from build123d import *

# Parameters (mm, degrees)
SKETCH_1_W               = 5
SKETCH_1_H               = 3.2
SKETCH_2_OUTSIDE_W       = 14.9
SKETCH_2_OUTSIDE_H       = 14.9
CUT_EXTRUDE_1_DEPTH      = 3.2
SKETCH_3_R               = 1.5
CUT_EXTRUDE_2_DEPTH      = 1
CUT_EXTRUDE_2_DEPTH_BACK = 4.2
CHAMFER_1_SIZE           = 0.4


with BuildPart() as part:
    # Эскиз1 → Повернуть1 (revolve)
    with BuildSketch(Plane(origin=(0, 0, 0), x_dir=(1, 0, 0), z_dir=(0, 1, 0))):
        with Locations((-2.5, 1.6)):
            Rectangle(SKETCH_1_W, SKETCH_1_H)
    revolve(axis=Axis((0, 0, 0), (0, 0, -1)))

    # Эскиз2 outside → Вырез-Вытянуть1 (cut)
    with BuildSketch(Plane.XY):
        Rectangle(SKETCH_2_OUTSIDE_W, SKETCH_2_OUTSIDE_H)
        Polygon((3, -1.732050808), (3, 1.732050808), (0, 3.464101615), (-3, 1.732050808), (-3, -1.732050808), (0, -3.464101615), align=None, mode=Mode.SUBTRACT)
    extrude(amount=-CUT_EXTRUDE_1_DEPTH, mode=Mode.SUBTRACT)

    # Эскиз3 → Вырез-Вытянуть2 (cut, two sides)
    with BuildSketch(Plane.XY) as cut_extrude_2_sk:
        Circle(SKETCH_3_R)
    extrude(amount=CUT_EXTRUDE_2_DEPTH, mode=Mode.SUBTRACT)
    extrude(cut_extrude_2_sk.sketch, amount=-CUT_EXTRUDE_2_DEPTH_BACK, mode=Mode.SUBTRACT)

    # Эскиз4 → Вырез-Повернуть1 (revolve, cut)
    with BuildSketch(Plane(origin=(0, 0, 0), x_dir=(0, 0, -1), z_dir=(1, 0, 0))):
        Polygon((0, 2.8), (0.383419246, 3.464101615), (0, 3.464101615), align=None)
        Polygon((3.2, 2.8), (2.816580754, 3.464101615), (3.2, 3.464101615), align=None)
    revolve(axis=Axis((0, 0, 0), (0, 0, -1)), mode=Mode.SUBTRACT)

    # Фаска1
    chamfer_1_edges = [part.edges().sort_by_distance(p)[0] for p in [
        (-1.5, 0, -3.2),
        (-1.5, 0, 0),
    ]]
    chamfer(chamfer_1_edges, length=CHAMFER_1_SIZE)


solid = part.part
Source: CAD feature listing. Evaluate the final solid. Frame: model axes, mm. Round coordinates to 2 decimals unless told otherwise and drop trailing zeros. Order: outer loops, then holes, each group sorted by start corner. A loop starts at its lowest first (then second) coordinate and runs counter-clockwise, first axis right, second up. Notation, with made-up numbers: (66, -21.75) - (104, -21.75) arc R18 cw to (104, -5.75) - close; hole circle Ø11 at (10, 21). An arc over 180 degrees is marked (long way). Use a Markdown table: item, result. Add a question column.
1. Line query: probe 1 along Y at (x, z) = (1.3, -2.85); probe 2 along Y at (x, z) = (-0.9, -0.2); probe 3 along X at (y, z) = (-1, -0.95). Output: solid intervals per line, ascending.
2. Section query A-A (y = 0). Return the cut outline in (x, z).
3. First-contact query: pin 1 (3.5 mm diameter, centred on x = 0, y = 0, fed in from +Z); pin 2 (1 mm diameter, centred on y = -2, z = -0.5, fed in from -X); pin 3 (1.5 mm diameter, centred on x = -1.5, z = -2.5, fed in from -Y). Flat tips, straight axial feed; report the tip coordinate or a pass-through.
4. Section query B-B (z = -1.95). Return the cut outline in (x, y).
5. Mould query, pull axis Y, two halves, no side actions, for faces 1 (the flat face through (-1, -2, 0)), 2 (the flat face through (-1.5, -2.6, -1.6)), 3 (the cylindrical face through (-1.5, 0.07, -1.58)). Classes: +Y half, -Y half, draft (parallel to the pull), parting line (faces both ways), or undercut.
Derived:
| question | item | result |
|---|---|---|
| 1 | probe 1 | -2.71 to -0.84, 0.84 to 2.71 |
| 1 | probe 2 | -2.94 to -1.44, 1.44 to 2.94 |
| 1 | probe 3 | -3 to -1.12, 1.12 to 3 |
| 2 | outline | (-3, -3.08) - (-2.8, -3.2) - (-1.9, -3.2) - (-1.5, -2.8) - (-1.5, -0.4) - (-1.9, 0) - (-2.8, 0) - (-3, -0.12) - close; (1.5, -2.8) - (1.9, -3.2) - (2.8, -3.2) - (3, -3.08) - (3, -0.12) - (2.8, 0) - (1.9, 0) - (1.5, -0.4) - close |
| 3 | pin 1 | z = -0.15 |
| 3 | pin 2 | x = -3 |
| 3 | pin 3 | y = -3.03 |
| 4 | outline | (-3, -1.73) - (0, -3.46) - (3, -1.73) - (3, 1.73) - (0, 3.46) - (-3, 1.73) - close; hole circle Ø3 at (0, 0) |
| 5 | face 1 | draft |
| 5 | face 2 | -Y half |
| 5 | face 3 | undercut |
